Check sheet for the modelled part. Datum: model origin and axes. Units: mm. A direction names the side the tool comes from. Round coordinates to 2 decimals unless told otherwise and drop trailing zeros. Loops run counter-clockwise (first coordinate to the right, second up) from the corner with the lowest first, then second, coordinate; pieces in that order, holes last. Notation, with made-up numbers: (34.25, -32.75) - (80.25, -32.75) arc R11 ccw to (80.25, -27.75) - close; hole circle Ø11 at (24.25, 13). An arc over 180 degrees is marked (long way). Put each result on its own line as item: value. Start each with the question number.
Item 1: Section check B-B, the plane x = 14. Record the cut outline in (y, z).
Item 2: Material ranges on line 1 along Y through (x, z) = (-30, 12.75); line 2 along Y through (x, z) = (42.25, 14.5); line 3 along X through (y, z) = (9, 14.5), recorded low to high.
Item 3: Section check C-C, the plane y = 4. Record the cut outline in (x, z).
Item 4: Draft check along Y on faces 5 (the cylindrical face through (47.72, 16.75, 1.23)), 6 (the cylindrical face through (43.9, -20.43, 10.1)), 7 (the flat face through (46, 0, 2.5)), 8 (the cylindrical face through (-43.24, -19.51, 12.57)). Enter one of: pulls with the +Y half, pulls with the -Y half, needs draft (parallel to the pull), parting line crosses it, or undercut.
Item 5: Tool access check on faces 1 (the flat face through (-42, -19, 7.5)), 2 (the flat face through (47.162, 19.463, 1.232)), 3 (the cylindrical face through (41.26, 19.51, 1.23)), 4 (the flat face through (44.5, 0, 10)). Record the directions out of +Z, -Z, +X, -X, +Y, -Y that give a thin tool (end or side, any length) a straight path to the whole face; none if there is none.
Item 6: Section check A-A, the plane z = 1.5. Record the cut outline in (x, y), and give its area (3 significant figures).
Item 7: Gauge pin test, flat ends, axial feed: pin 1 Ø2 at (x, y) = (42.25, -18.75) entering from +Z; pin 2 Ø6 at (y, z) = (11, 9) entering from +X; pin 3 Ø6 at (x, y) = (-22.5, -11) entering from +Z. Record the tip position at first contact, or that the pin passes through.
Autodesk Fusion 360 part; units mm, degrees
sketch "Sketch1" plane through (0, 0, 0) normal (0, 0, 1) x (1, 0, 0)
  line L0 (37.5, 17.5) -> (-37.5, 17.5)
  line L1 (-37.5, 17.5) -> (-37.5, -17.5)
  line L2 (-37.5, -17.5) -> (37.5, -17.5)
  line L3 (37.5, -17.5) -> (37.5, 17.5)
  line L4 (37.5, 17.5) -> (-37.5, -17.5) construction
  line L5 (-37.5, 17.5) -> (37.5, -17.5) construction
  line L6 (44.5, 21) -> (-44.5, 21)
  line L7 (-44.5, 21) -> (-44.5, -21)
  line L8 (-44.5, -21) -> (44.5, -21)
  line L9 (44.5, -21) -> (44.5, 21)
  line L10 (44.5, 21) -> (-44.5, -21) construction
  line L11 (-44.5, 21) -> (44.5, -21) construction
  line L12 (0, 2.5) -> (0, 20)
  line L13 (44.5, -21) -> (50.75, -17.3916)
  line L14 (50.75, -17.3916) -> (50.75, 17.3916)
  line L15 (50.75, 17.3916) -> (44.5, 21)
  line L16 (46.5, 15.5) -> (46.5, -15.5)
  arc A0 (46.5, -15.5) -> (49, -15.5) centre (47.75, -15.5) ccw
  line L17 (49, -15.5) -> (49, 15.5)
  arc A1 (49, 15.5) -> (46.5, 15.5) centre (47.75, 15.5) ccw
  line L18 (47.75, 15.5) -> (47.75, -15.5) construction
  arc A2 (-49, -15.5) -> (-46.5, -15.5) centre (-47.75, -15.5) ccw
  line L19 (-46.5, 15.5) -> (-46.5, -15.5)
  line L20 (-49, -15.5) -> (-49, 15.5)
  arc A3 (-46.5, 15.5) -> (-49, 15.5) centre (-47.75, 15.5) ccw
  line L21 (-50.75, 17.3916) -> (-44.5, 21)
  line L22 (-50.75, -17.3916) -> (-50.75, 17.3916)
  line L23 (-44.5, -21) -> (-50.75, -17.3916)
  line L24 (38.5, 18.5) -> (-38.5, 18.5)
  line L25 (-38.5, 18.5) -> (-38.5, -18.5)
  line L26 (-38.5, -18.5) -> (38.5, -18.5)
  line L27 (38.5, -18.5) -> (38.5, 18.5)
  line L28 (38.5, 18.5) -> (-38.5, -18.5) construction
  line L29 (-38.5, 18.5) -> (38.5, -18.5) construction
  line L30 (40, 20) -> (-40, 20)
  line L31 (-40, 20) -> (-40, -20)
  line L32 (-40, -20) -> (40, -20)
  line L33 (40, -20) -> (40, 20)
  line L34 (40, 20) -> (-40, -20) construction
  line L35 (-40, 20) -> (40, -20) construction
  circle A4 centre (42.25, 18.75) radius 1.25
  circle A5 centre (-42.25, 18.75) radius 1.25
  line L36 (20, 0) -> (2.5, 0)
  circle A6 centre (42.25, -18.75) radius 1.25
  circle A7 centre (-42.25, -18.75) radius 1.25
  line L37 (-107, 0) -> (107, 0)
  point P0 (47.75, 0)
  dimension "d1" = 35
  dimension "d3" = 75
  dimension "d26" = 120
  dimension "d46" = 3.5
  dimension "d47" = 1
  dimension "d48" = 1
  dimension "d49" = 1
  dimension "d51" = 1.5
  dimension "d52" = 89
  dimension "d53" = 2.5
  dimension "d54" = 2.25
  dimension "d55" = 2.25
  dimension "d56" = 2.5
  dimension "d57" = 6.25
  dimension "d66" = 2
  dimension "d67" = 31
extrude "Extrude2" add sketch "Sketch1" along normal blind 2.5 contours L0 L1 L3 L36 L37 | L0 L3 L12 L24 L27 L37 | L0 L1 L12 L24 L25 L37 | L1 L2 L3 L25 L26 L27 L37 | L1 L2 L3 L36 L37 | L12 L24 L25 L30 L31 L37 | L12 L24 L27 L30 L33 L37 | L25 L26 L27 L31 L32 L33 L37 | L6 L7 L9 L30 L31 L33 L37 | L7 L8 L9 L31 L32 L33 L37 | L9 L13 L14 L16 A0 L17 L37 | L9 L14 L15 L16 L17 A1 L37 | L7 L19 L20 A3 L21 L22 L37 | L7 A2 L19 L20 L22 L23 L37
extrude "Extrude14" add sketch "Sketch1" along normal blind 15 from surface at 2.5 contours L0 L3 L12 L24 L27 L37 | L0 L1 L12 L24 L25 L37 | L1 L2 L3 L25 L26 L27 L37 | L12 L24 L25 L30 L31 L37 | L12 L24 L27 L30 L33 L37 | L25 L26 L27 L31 L32 L33 L37 | L6 L7 L9 L30 L31 L33 L37 | L7 L8 L9 L31 L32 L33 L37 | A4 | A5 | A6 | A7
extrude "Extrude15" cut sketch "Sketch1" against normal blind 5 from surface at 17.5 contours L12 L24 L25 L30 L31 L37 | L12 L24 L27 L30 L33 L37 | L25 L26 L27 L31 L32 L33 L37
extrude "Extrude16" cut sketch "Sketch1" against normal blind 10 from surface at 17.5 contours A4 | A5 | A6 | A7
fillet "Fillet5" radius 2 20 edges at (-50.75, -17.3916, 1.25) (-44.5, -21, 10) (-50.75, 17.3916, 1.25) (-44.5, 21, 10) (-38.5, 18.5, 15) (-40, 20, 15) (-37.5, 17.5, 10) (-37.5, -17.5, 10) (-38.5, -18.5, 15) (-40, -20, 15) (37.5, 17.5, 10) (40, 20, 15) (37.5, -17.5, 10) (38.5, -18.5, 15) (40, -20, 15) (44.5, -21, 10) (50.75, -17.3916, 1.25) (38.5, 18.5, 15) (44.5, 21, 10) (50.75, 17.3916, 1.25)
equation "d48 = d47"
equation "d49 = d47"
equation "d51 = d46 - 2 * d47"
equation "d52 = d3 + 2 * d46 + 2 * d47 + 2 * d53"
equation "d54 = d47 + 0.5 * d53"
equation "d55 = d47 + 0.5 * d53"
equation "d56 = d53"
equation "d57 = d54 + 4 * d47"
equation "d66 = 2 * d47"
equation "d67 = d1 - 4 * d47"
equation "d80 = d7"
equation "d83 = d7 + d81"
equation "d86 = d7 + d81"
Check result:
1. outline: (-21, 0) - (21, 0) - (21, 17.5) - (20, 17.5) - (20, 12.5) - (18.5, 12.5) - (18.5, 17.5) - (17.5, 17.5) - (17.5, 2.5) - (-17.5, 2.5) - (-17.5, 17.5) - (-18.5, 17.5) - (-18.5, 12.5) - (-20, 12.5) - (-20, 17.5) - (-21, 17.5) - close
2. line 1: -21 to -20, -18.5 to -17.5, 17.5 to 18.5, 20 to 21
2. line 2: -21 to -20, -17.5 to 17.5, 20 to 21
2. line 3: -44.5 to -40, -38.5 to -37.5, 37.5 to 38.5, 40 to 44.5
3. outline: (-50.75, 0) - (-49, 0) - (-49, 2.5) - (-50.75, 2.5) - close; (-46.5, 0) - (46.5, 0) - (46.5, 2.5) - (44.5, 2.5) - (44.5, 17.5) - (40, 17.5) - (40, 12.5) - (38.5, 12.5) - (38.5, 17.5) - (37.5, 17.5) - (37.5, 2.5) - (-37.5, 2.5) - (-37.5, 17.5) - (-38.5, 17.5) - (-38.5, 12.5) - (-40, 12.5) - (-40, 17.5) - (-44.5, 17.5) - (-44.5, 2.5) - (-46.5, 2.5) - close; (49, 0) - (50.75, 0) - (50.75, 2.5) - (49, 2.5) - close
4. face 5: undercut
4. face 6: pulls with the -Y half
4. face 7: needs draft
4. face 8: undercut
5. face 1: +Z
5. face 2: +Z, -Z, +X, +Y
5. face 3: -Z
5. face 4: +Z, +X, +Y, -Y
6. outline: (-50.75, -16.24) arc R2 ccw to (-49.75, -17.97) - (-44.5, -21) - (44.5, -21) - (49.75, -17.97) arc R2 ccw to (50.75, -16.24) - (50.75, 16.24) arc R2 ccw to (49.75, 17.97) - (44.5, 21) - (-44.5, 21) - (-49.75, 17.97) arc R2 ccw to (-50.75, 16.24) - close; hole (-49, -15.5) arc R1.25 ccw to (-46.5, -15.5) - (-46.5, 15.5) arc R1.25 ccw to (-49, 15.5) - close; hole circle Ø2.5 at (-42.25, -18.75); hole circle Ø2.5 at (-42.25, 18.75); hole circle Ø2.5 at (42.25, -18.75); hole circle Ø2.5 at (42.25, 18.75); hole (46.5, -15.5) arc R1.25 ccw to (49, -15.5) - (49, 15.5) arc R1.25 ccw to (46.5, 15.5) - close
6. area: 4,030 mm²
7. pin 1: z = 7.5
7. pin 2: x = 44.5
7. pin 3: z = 2.5
